```python
from build123d import *

# Parameters (mm, degrees)
SKETCH_1_W                   = 150
SKETCH_1_H                   = 40
BASEPLATE_DEPTH              = 10
VERTBOSS_DEPTH               = 10
SKETCH_3_W                   = 40
SKETCH_3_H                   = 3
BOTTOMSOLT_DEPTH             = 165.69669092
HOLE_WIZARD_M8_1_D           = 9
HOLE_WIZARD_M8_1_CBORE_D     = 18.01
HOLE_WIZARD_M8_1_CBORE_DEPTH = 5.68
HOLE_WIZARD_7_0_7_1_D        = 7
FILLET_1_R                   = 8
FILLET_2_R                   = 3


with BuildPart() as part:
    # 草圖1 → BasePlate (new body)
    with BuildSketch(Plane(origin=(0, 0, 0), x_dir=(1, 0, 0), z_dir=(0, 1, 0))):
        with Locations((75, 20)):
            Rectangle(SKETCH_1_W, SKETCH_1_H)
    extrude(amount=BASEPLATE_DEPTH)

    # 草圖2 → VertBoss (add)
    with BuildSketch(Plane.XY):
        with BuildLine():
            Line((30, 0), (30, 35))
            ThreePointArc((30, 35), (50, 55), (70, 35))
            Line((70, 35), (70, 0))
            Line((70, 0), (30, 0))
        make_face()
    extrude(amount=-VERTBOSS_DEPTH)

    # 草圖3 → BottomSolt (cut, through all)
    with BuildSketch(Plane.XY):
        with Locations((50, 1.5)):
            Rectangle(SKETCH_3_W, SKETCH_3_H)
    extrude(amount=-BOTTOMSOLT_DEPTH, mode=Mode.SUBTRACT)

    # M8 六角頭螺栓的柱孔1 (through all)
    with Locations(Plane.XY):
        with Locations((50, 35)):
            CounterBoreHole(HOLE_WIZARD_M8_1_D / 2, HOLE_WIZARD_M8_1_CBORE_D / 2, HOLE_WIZARD_M8_1_CBORE_DEPTH)

    # Ø7.0 (7) 直徑孔1 (through all)
    with Locations(Plane(origin=(0, 10, 0), x_dir=(1, 0, 0), z_dir=(0, 1, 0))):
        with Locations((15, 30), (135, 30)):
            Hole(HOLE_WIZARD_7_0_7_1_D / 2)

    # 圓角1
    # the kernel refuses this fillet: 8 mm, written as the material it adds along each edge
    with BuildSketch(Plane(origin=(70, 3, 0), x_dir=(-1, 0, 0), z_dir=(0, 0, -1))) as fillet_1_piece_1:
        with BuildLine():
            CenterArc((6.244997998, -8), FILLET_1_R, 90, 51.317812547)
            Line((0, -3), (0, 0))
            Line((0, 0), (6.244997998, 0))
        make_face()
    extrude(amount=40)
    with BuildSketch(Plane(origin=(30, 3, 0), x_dir=(0, -1, 0), z_dir=(0, 0, -1))) as fillet_1_piece_2:
        with BuildLine():
            CenterArc((8, -6.244997998), FILLET_1_R, 128.682187453, 51.317812547)
            Line((0, -6.244997998), (0, 0))
            Line((0, 0), (3, 0))
        make_face()
    extrude(amount=40)
    # the kernel refuses this fillet: 8 mm, written as the material it takes off along each edge
    with BuildSketch(Plane(origin=(0, -20, 0), x_dir=(1, 0, 0), z_dir=(0, 1, 0)), Plane(origin=(0, -20, -40), x_dir=(0, 0, 1), z_dir=(0, 1, 0))) as fillet_1_2_piece_1:
        with BuildLine():
            CenterArc((FILLET_1_R, FILLET_1_R), FILLET_1_R, 180, 90)
            Line((0, FILLET_1_R), (0, 0))
            Line((0, 0), (FILLET_1_R, 0))
        make_face()
    extrude(amount=50, mode=Mode.SUBTRACT)
    with BuildSketch(Plane(origin=(150, -20, 0), x_dir=(-1, 0, 0), z_dir=(0, 1, 0)), Plane(origin=(150, -20, -40), x_dir=(0, 0, 1), z_dir=(0, 1, 0))) as fillet_1_2_piece_2:
        with BuildLine():
            CenterArc((FILLET_1_R, -FILLET_1_R), FILLET_1_R, 90, 90)
            Line((0, -FILLET_1_R), (0, 0))
            Line((0, 0), (FILLET_1_R, 0))
        make_face()
    extrude(amount=50, mode=Mode.SUBTRACT)

    # 圓角2
    fillet_2_edges = [part.edges().sort_by_distance(p)[0] for p in [
        (106, 10, 0),
        (30, 22.5, -10),
        (70, 22.5, -10),
        (30, 22.5, 0),
        (70, 22.5, 0),
        (50, 55, 0),
        (30, 10, -5),
        (50, 55, -10),
        (70, 10, -5),
        (50, 10, -10),
        (19, 10, 0),
        (0, 10, -20),
        (150, 10, -20),
        (75, 10, -40),
        (147.656854249, 10, -37.656854249),
        (147.656854249, 10, -2.343145751),
        (2.343145751, 10, -37.656854249),
        (2.343145751, 10, -2.343145751),
    ]]
    fillet(fillet_2_edges, radius=FILLET_2_R)


solid = part.part
```
Check sheet for the modelled part. Datum: model origin and axes. Units: mm. A direction names the side the tool comes from. Round coordinates to 2 decimals unless told otherwise and drop trailing zeros. Order: outer loops, then holes, each group sorted by start corner. A loop starts at its lowest first (then second) coordinate and runs counter-clockwise, first axis right, second up. Notation, with made-up numbers: (75.25, 82.5) -> (107.25, 82.5) arc R17 ccw to (107.25, 100.5) -> close; hole circle Ø8 at (-18, 12.5). An arc over 180 degrees is marked (long way). One line per item, written item: value. Start each with the question number.
Q1. Set-up check for faces 5 (the face through (107.98, 9.1, -0.86)), 6 (the face through (58.32, 31.55, -2.8)), 7 (the face through (30.86, 24.15, -9.1)): record each of +Z, -Z, +X, -X, +Y, -Y from which the full face is reachable in a straight line by a thin tool's end or side.
Q2. Gauge pin test, flat ends, axial feed: pin 1 Ø22 at (x, z) = (44, -12.5) entering from -Y; pin 2 Ø10 at (x, y) = (62, 21) entering from -Z; pin 3 Ø11 at (x, z) = (135, -30) entering from -Y; pin 4 Ø1.5 at (y, z) = (36.5, -12.5) entering from +X. Record the tip position at first contact, or that the pin passes through.
Q3. Cross-section at B-B (z = -30). Record the boundary of the cut face in (x, y) (3 decimals), and give its area (3 significant figures).
Q4. Cross-section at D-D (z = -21.5). Record the boundary of the cut face in (x, y) (3 decimals), and give its area (3 significant figures).
Q5. Mould release check, pull along X, two halves, no side actions. Record for faces 1 (the face through (67.174, 2.233, -19.72)), 2 (the face through (0.86, 9.1, -19.83)), 3 (the face through (131.66, 4.93, -31.05)), 4 (the face through (149.14, 9.1, -20.17)): pulls with the +X half, pulls with the -X half, needs draft (parallel to the pull), parting line crosses it, or undercut.
Q6. Cross-section at A-A (x = 50). Record the boundary of the cut face in (y, z) (3 decimals).
Q7. Thickness scan on line 1 (X direction, y = 3.5, z = -30); line 2 (Z direction, x = 135, y = 7); line 3 (Y direction, x = 83, z = -11). Record the ranges inside material, lowest first.
Q8. Cross-section at C-C (x = 15). Record the boundary of the cut face in (y, z).
Completed:
1. face 5: +Z, +X, +Y
1. face 6: +Z
1. face 7: -Z, -X, +Y
2. pin 1: stops at y = 2.31
2. pin 2: stops at z = -10
2. pin 3: stops at y = 0
2. pin 4: passes through
3. outline: (0, 0) -> (11.5, 0) -> (11.5, 10) -> (3, 10) arc R3 ccw to (0, 7) -> close; (18.5, 0) -> (30, 0) arc R8 cw to (36.245, 3) -> (63.755, 3) arc R8 cw to (70, 0) -> (131.5, 0) -> (131.5, 10) -> (18.5, 10) -> close; (138.5, 0) -> (150, 0) -> (150, 7) arc R3 ccw to (147, 10) -> (138.5, 10) -> close
3. area: 1,250 mm²
4. outline: (0, 0) -> (30, 0) arc R8 cw to (36.245, 3) -> (63.755, 3) arc R8 cw to (70, 0) -> (150, 0) -> (150, 7) arc R3 ccw to (147, 10) -> (3, 10) arc R3 ccw to (0, 7) -> close
4. area: 1,390 mm²
5. face 1: undercut
5. face 2: pulls with the -X half
5. face 3: undercut
5. face 4: pulls with the +X half
6. outline: (3, -40) -> (7, -40) arc R3 ccw to (10, -37) -> (10, -13) arc R3 cw to (13, -10) -> (30.5, -10) -> (30.5, -5.68) -> (25.995, -5.68) -> (25.995, 0) -> (3, 0) -> close; (39.5, -10) -> (52, -10) arc R3 ccw to (55, -7) -> (55, -3) arc R3 ccw to (52, 0) -> (44.005, 0) -> (44.005, -5.68) -> (39.5, -5.68) -> close
7. line 1: x = 0 to 11.5, 18.5 to 131.5, 138.5 to 150
7. line 2: z = -40 to -33.5, -26.5 to 0
7. line 3: y = 0 to 10
8. outline: (0, -40) -> (7, -40) arc R3 ccw to (10, -37) -> (10, -33.5) -> (0, -33.5) -> close; (0, -26.5) -> (10, -26.5) -> (10, -3) arc R3 ccw to (7, 0) -> (0, 0) -> close
